Here's the drawing with two shaded views (mm, measured from the low corner). I have some questions. Coordinates: 2 decimals unless noted, no trailing zeros. Loops run counter-clockwise (first coordinate to the right, second up) from the corner with the lowest first, then second, coordinate; pieces in that order, holes last. Notation, with made-up numbers: (4.5, 3) - (21.5, 3) arc R28 ccw to (21.5, 35) - close; hole circle Ø10 at (-16.75, -40). An arc over 180 degrees is marked (long way). One line per item, written item: value. Start each with the question number.
(1) If we section it at D-D on x = 20.25: Write out the boundary of the cut face in (y, z).
(2) If I drill on line 1 along Y through (x, z) = (15, 1.05); line 2 along X through (y, z) = (8, 1.05); line 3 along Z through (x, y) = (15, 23.9), over which ranges is the centre line in solid material (lowest first)? Write a range as from..to.
(3) I'm going to push flat-ended pins straight in: P1, Ø3, axis at x = 19.5, y = 6, coming from the +Z side; P2, Ø2, axis at x = 16.5, z = 10, coming from the -Y side; P3, Ø5, axis at x = 15, z = 17, coming from the -Y side. Where does each tip first touch, or does it pass through?
(4) If we mould it in two halves opening along Y, with no side actions, what happens to the marked faces 1, 2 and 3? For each: pulls with the +Y half, pulls with the -Y half, needs draft (parallel to the pull), parting line crosses it, or undercut.
(5) If we section it at A-A on x = 15: Write out the boundary of the cut face in (y, z), then the cut area to 4 significant figures.
(6) If we section it at B-B on y = 8: Write out the boundary of the cut face in (x, z), then the cut area to 4 significant figures.
(7) If we section it at C-C on z = 17: Write out the boundary of the cut face in (x, y), then the cut area to 4 significant figures.
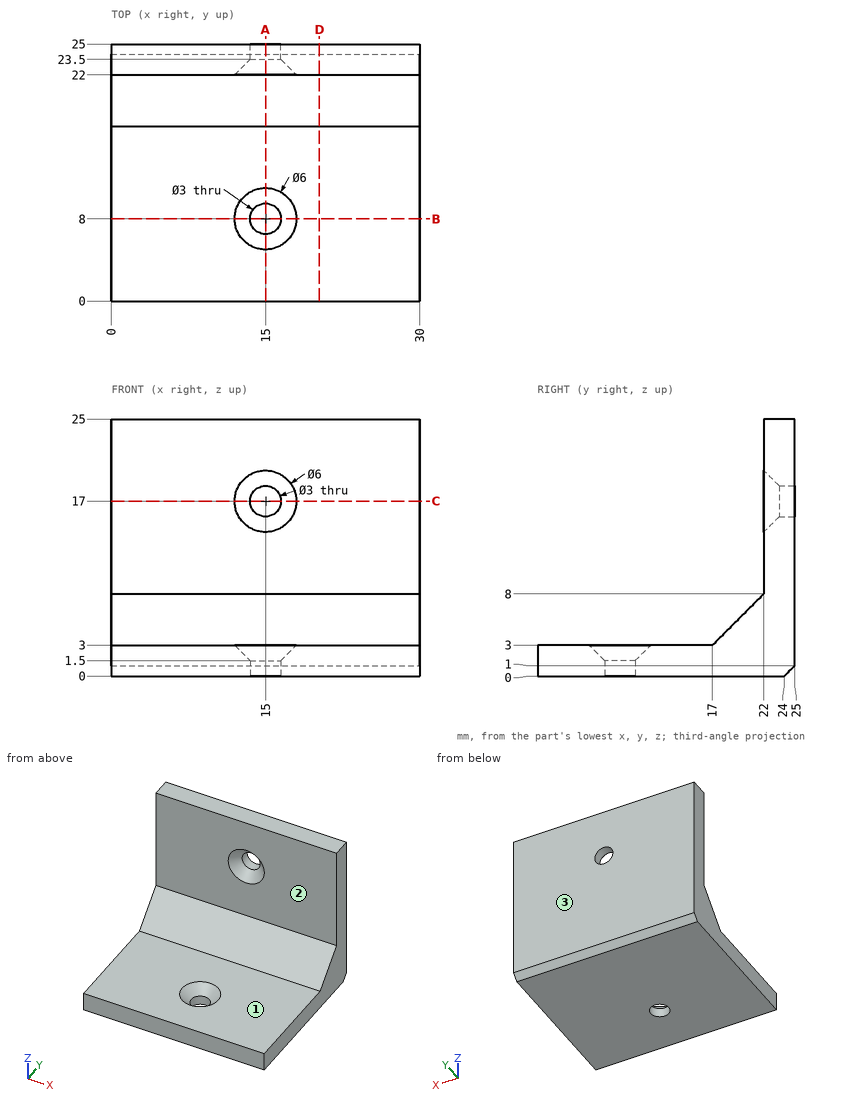
Values:
1. outline: (0, 0) - (24, 0) - (25, 1) - (25, 25) - (22, 25) - (22, 8) - (17, 3) - (0, 3) - close
2. line 1: y = 0..6.5, 9.5..25
2. line 2: x = 0..13.5, 16.5..30
2. line 3: z = 0..15.5, 18.5..25
3. P1: stops at z = 3
3. P2: stops at y = 22
3. P3: stops at y = 22.5
4. face 1: needs draft
4. face 2: pulls with the -Y half
4. face 3: pulls with the +Y half
5. outline: (0, 0) - (6.5, 0) - (6.5, 1.5) - (5, 3) - (0, 3) - close; (9.5, 0) - (24, 0) - (25, 1) - (25, 15.5) - (23.5, 15.5) - (22, 14) - (22, 8) - (17, 3) - (11, 3) - (9.5, 1.5) - close; (22, 20) - (23.5, 18.5) - (25, 18.5) - (25, 25) - (22, 25) - close
5. area: 130.5 mm2
6. outline: (0, 0) - (13.5, 0) - (13.5, 1.5) - (12, 3) - (0, 3) - close; (16.5, 0) - (30, 0) - (30, 3) - (18, 3) - (16.5, 1.5) - close
6. area: 78.75 mm2
7. outline: (0, 22) - (12, 22) - (13.5, 23.5) - (13.5, 25) - (0, 25) - close; (16.5, 23.5) - (18, 22) - (30, 22) - (30, 25) - (16.5, 25) - close
7. area: 78.75 mm2
